Check sheet for the modelled part. Datum: model origin and axes. Units: mm. Face numbers are marked on the shaded views. A direction names the side the tool comes from. Round coordinates to 2 decimals unless told otherwise and drop trailing zeros. Loops run counter-clockwise (first coordinate to the right, second up) from the corner with the lowest first, then second, coordinate; pieces in that order, holes last. Notation, with made-up numbers: (-5, 5) - (36, 5) arc R12 cw to (36, 21) - close; hole circle Ø5 at (70.5, -34). An arc over 180 degrees is marked (long way). Answer in a Markdown table with one row per item. Add a question column.
(1) Cross-section at C-C on y = 12. Enter the section's corners in (x, z) (1 decimal).
(2) Thickness scan on line 1 along Z through (x, y) = (19, 9.5) (3 decimals); line 2 along X through (y, z) = (15, -50); line 3 along X through (y, z) = (7, -43). Record the ranges inside material, lowest first.
(3) Cross-section at B-B on x = 16.5. Enter the section's corners in (y, z) (3 decimals).
(4) Cross-section at D-D on z = -6. Enter the section's corners in (x, y).
(5) Cross-section at A-A on z = -40.5. Enter the section's corners in (x, y).
(6) Gauge pin test, flat ends, axial feed: pin 1 (5 mm diameter, centred on x = 26.5, y = 4.5, fed in from +Z); pin 2 (6.5 mm diameter, centred on y = 14.5, z = -47, fed in from +X); pin 3 (6.5 mm diameter, centred on y = 4.445, z = -7.62, fed in from +X); pin 4 (4 mm diameter, centred on y = 4, z = -37, fed in from +X). Record the tip position at first contact, or that the pin passes through.
(7) Mould release check, pull along Y, two halves, no side actions. Record for the marked faces 3, 4, 5 and 6: +Y half, -Y half, draft (parallel to the pull), parting line (faces both ways), or undercut.
(8) Access from +Z, -Z, +X, -X, +Y, -Y to the whole of each face (thin tool, end or side, straight path). Record for the marked faces 1 and 2.
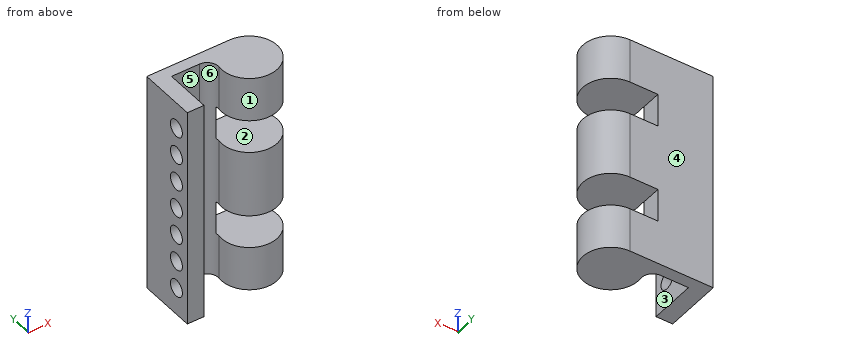
Autodesk Inventor part; units mm, degrees
ref_plane "YZ Plane" through (0, 0, 0) normal (1, 0, 0) x (0, 1, 0)
ref_plane "XZ Plane" through (0, 0, 0) normal (0, 1, 0) x (-1, 0, 0)
ref_plane "XY Plane" through (0, 0, 0) normal (0, 0, 1) x (1, 0, 0)
sketch "Sketch1" plane through (0, 0, 0) normal (1, 0, 0) x (0, 1, 0)
  line L0 (0, 0) -> (16.51, 0)
  line L1 (16.51, 0) -> (16.51, -63.5)
  line L2 (16.51, -63.5) -> (0, -63.5)
  line L3 (0, -63.5) -> (0, 0)
  circle A0 centre (4.445, -7.62) radius 2.4329
  circle A1 centre (4.445, -15.6185) radius 2.4329
  circle A2 centre (4.445, -23.6169) radius 2.4329
  circle A3 centre (4.445, -31.6154) radius 2.4329
  circle A4 centre (4.445, -39.6138) radius 2.4329
  circle A5 centre (4.445, -47.6123) radius 2.4329
  circle A6 centre (4.445, -55.6108) radius 2.4329
  dimension "d0" = 63.5
  dimension "d1" = 16.51
  dimension "d6" = 7.9985
  dimension "d11" = 7.62
extrude "Extrusion1" add sketch "Sketch1" along normal blind 4.7625
sketch "Sketch2" plane through (4.7625, 0, 0) normal (1, 0, 0) x (0, 0, -1)
  line L0 (63.5, 16.51) -> (0, 16.51)
  line L1 (63.5, 0) -> (63.5, 16.51)
  line L2 (0, 16.51) -> (63.5, 16.51)
  line L3 (63.5, 16.51) -> (63.5, 13.208)
  line L4 (63.5, 13.208) -> (0, 13.208)
  line L5 (0, 13.208) -> (0, 16.51)
  point P0 (0, 0)
  dimension "d14" = 3.302
extrude "Extrusion2" add sketch "Sketch2" along normal blind 1.016
sketch "Sketch3" plane through (0, 0, 0) normal (0, 0, 1) x (1, 0, 0)
  line L0 (5.7785, 16.51) -> (5.7785, 13.208)
  arc A0 (15.8804, 9.6157) -> (23.749, 16.51) centre (23.749, 8.5725) ccw
  line L1 (0, 16.51) -> (0, 0)
  line L2 (5.7785, 16.51) -> (23.749, 16.51)
  line L3 (4.7625, 13.208) -> (5.7785, 13.208)
  line L4 (5.7785, 13.208) -> (12.7329, 13.208)
  arc A1 (15.8804, 9.6157) -> (12.7329, 13.208) centre (12.7329, 10.033) ccw
  point P0 (17.3057, 13.208)
  point P1 (9.5258, 13.208)
  dimension "d17" = 23.749
  dimension "d18" = 15.875
  dimension "d19" = 3.175
extrude "Extrusion3" add sketch "Sketch3" against normal blind 63.5
sketch "Sketch4" plane through (0, 16.51, 0) normal (0, 1, 0) x (1, 0, 0)
  line L0 (31.6865, 0) -> (31.6865, 63.5)
  line L1 (31.6865, 0) -> (31.6865, 83.2403)
  point P0 (0, 0)
ref_plane "Work Plane1" through (55.5625, 0, 0) normal (1, 0, 0) x (0, 0, -1)
sketch "Sketch6" plane through (0, 16.51, 0) normal (0, 1, 0) x (1, 0, 0)
  line L0 (31.6865, 0) -> (31.6865, 63.5)
  line L1 (15.8115, 50.8) -> (31.6865, 50.8)
  line L2 (31.6865, 50.8) -> (31.6865, 41.275)
  line L3 (31.6865, 41.275) -> (15.8115, 41.275)
  line L4 (15.8115, 41.275) -> (15.8115, 50.8)
  line L5 (31.6865, 63.5) -> (15.8115, 63.5)
  line L6 (15.8115, 22.225) -> (31.6865, 22.225)
  line L7 (31.6865, 22.225) -> (31.6865, 12.7)
  line L8 (31.6865, 12.7) -> (15.8115, 12.7)
  line L9 (15.8115, 12.7) -> (15.8115, 22.225)
  line L10 (15.8115, 0) -> (31.6865, 0)
  point P0 (0, 0)
  point P1 (15.8804, 63.5)
  point P2 (15.8804, 0)
  dimension "d26" = 9.525
  dimension "d27" = 12.7
  dimension "d28" = 9.525
  dimension "d29" = 12.7
  dimension "d32" = 15.875
  dimension "d33" = 15.875
extrude "Extrusion4" cut sketch "Sketch6" against normal through all
properties part number "knuckle plate hinge"
Answers:
| question | item | result |
|---|---|---|
| 1 | outline | (0, -63.5) - (4.8, -63.5) - (4.8, 0) - (0, 0) - close; (15.2, -63.5) - (30.9, -63.5) - (30.9, -50.8) - (15.8, -50.8) - (15.8, -41.3) - (30.9, -41.3) - (30.9, -22.2) - (15.8, -22.2) - (15.8, -12.7) - (30.9, -12.7) - (30.9, 0) - (15.2, 0) - close |
| 2 | line 1 | z = -63.5 to -50.8, -41.275 to -22.225, -12.7 to 0 |
| 2 | line 2 | x = 0 to 15.81 |
| 2 | line 3 | x = 0 to 4.76 |
| 3 | outline | (5.339, -63.5) - (16.51, -63.5) - (16.51, -50.8) - (5.339, -50.8) - close; (5.339, -41.275) - (16.51, -41.275) - (16.51, -22.225) - (5.339, -22.225) - close; (5.339, -12.7) - (16.51, -12.7) - (16.51, 0) - (5.339, 0) - close |
| 4 | outline | (0, 0) - (4.76, 0) - (4.76, 2.63) - (0, 2.63) - close; (0, 6.26) - (4.76, 6.26) - (4.76, 13.21) - (12.73, 13.21) arc R3.17 cw to (15.88, 9.62) arc R7.94 ccw (long way) to (23.75, 16.51) - (0, 16.51) - close |
| 5 | outline | (0, 0) - (4.76, 0) - (4.76, 2.18) - (0, 2.18) - close; (0, 6.71) - (4.76, 6.71) - (4.76, 13.21) - (12.73, 13.21) arc R3.17 cw to (15.88, 9.62) arc R7.94 ccw (long way) to (23.75, 16.51) - (0, 16.51) - close |
| 6 | pin 1 | stops at z = 0 |
| 6 | pin 2 | stops at x = 15.81 |
| 6 | pin 3 | stops at x = 31.64 |
| 6 | pin 4 | stops at x = 31.26 |
| 7 | face 3 | draft |
| 7 | face 4 | +Y half |
| 7 | face 5 | -Y half |
| 7 | face 6 | undercut |
| 8 | face 1 | +Z, -Z |
| 8 | face 2 | +X, +Y, -Y |
